Geometry check sheet. Reference: the model listing, model coordinates, mm. A direction names the side the tool comes from. Coordinates: 2 decimals unless noted, no trailing zeros. Order: outer loops, then holes, each group sorted by start corner. A loop starts at its lowest first (then second) coordinate and runs counter-clockwise, first axis right, second up. Notation, with made-up numbers: (5.5, -32) - (21.5, -32) arc R23 ccw to (21.5, -15) - close; hole circle Ø5 at (-37, -9). An arc over 180 degrees is marked (long way). Return JSON: item names as keys, results as strings. Group by question number.
Item 1: Gauge pin test, flat ends, axial feed: pin 1 (4 mm diameter, centred on y = -27, z = 74.5, fed in from +X); pin 2 (0.8 mm diameter, centred on x = -0.5, z = 22.5, fed in from -Y); pin 3 (1 mm diameter, centred on x = -36, z = 43, fed in from -Y). Record the tip position at first contact, or that the pin passes through.
Item 2: Section check B-B on z = 7. Enter the section's corners in (x, y).
Item 3: Scan lines: probe 1 along Z at (x, y) = (-48, -27); probe 2 along X at (y, z) = (-7.5, 62.5); probe 3 along X at (y, z) = (-30, 30.5). Record each from-to range of solid material in increasing order.
Item 4: Tool access check on faces 1 (the cylindrical face through (-2.1, -2.07, 39.44)), 2 (the flat face through (-1, -21.5, 39)), 3 (the flat face through (-28, -1, 0)). Record the directions out of +Z, -Z, +X, -X, +Y, -Y that give a thin tool (end or side, any length) a straight path to the whole face; none if there is none.
Item 5: Section check A-A on y = -16. Enter the section's corners in (x, z).
Item 6: Draft check along Z on faces 4 (the flat face through (-28, -1, 80)), 5 (the cylindrical face through (-48, -25, 7)), 6 (the flat face through (-25, -1.5, 39)). Enter one of: pulls with the +Z half, pulls with the -Z half, needs draft (parallel to the pull), parting line crosses it, or undercut.
Item 7: Section check D-D on z = 25.5. Enter the section's corners in (x, y).
Item 8: Section check C-C on y = -25.5. Enter the section's corners in (x, z).
from build123d import *

# Parameters (mm, degrees)
F1_DEPTH = 80
F2_R     = 2.5
F3_DEPTH = 1.5


with BuildPart() as f1:
    # F0 (on Top) → F1 (new body)
    with BuildSketch(Plane.XY):
        with BuildLine():
            ThreePointArc((0, -2), (-0.585786, -0.585786), (-2, 0))
            Line((-2, 0), (-47, 0))
            ThreePointArc((-47, 0), (-48.414214, -0.585786), (-49, -2))
            Line((-49, -2), (-49, -31.5))
            Line((-49, -31.5), (-47.5, -31.5))
            Line((-47.5, -31.5), (-47.5, -3.5))
            ThreePointArc((-47.5, -3.5), (-46.914214, -2.085786), (-45.5, -1.5))
            Line((-45.5, -1.5), (-3.5, -1.5))
            ThreePointArc((-3.5, -1.5), (-2.085786, -2.085786), (-1.5, -3.5))
            Line((-1.5, -3.5), (-1.5, -21.5))
            Line((-1.5, -21.5), (0, -21.5))
            Line((0, -21.5), (0, -2))
        make_face()
    extrude(amount=F1_DEPTH)

    # F2 (on face) → F3 (cut, through all)
    with BuildSketch(Plane(origin=(-49, 0, 0), x_dir=(0, -1, 0), z_dir=(-1, 0, 0))):
        with Locations((27, 5.5)):
            Circle(F2_R)
        with Locations((27, 74.5)):
            Circle(F2_R)
    extrude(amount=-F3_DEPTH, mode=Mode.SUBTRACT)


solid = f1.part
Computed:
{
 "1": {"pin 1": "passes through", "pin 2": "stops at y = -21.5", "pin 3": "stops at y = -1.5"},
 "2": {"outline": "(-49, -31.5) - (-47.5, -31.5) - (-47.5, -29) - (-49, -29) - close; (-49, -25) - (-47.5, -25) - (-47.5, -3.5) arc R2 cw to (-45.5, -1.5) - (-3.5, -1.5) arc R2 cw to (-1.5, -3.5) - (-1.5, -21.5) - (0, -21.5) - (0, -2) arc R2 ccw to (-2, 0) - (-47, 0) arc R2 ccw to (-49, -2) - close"},
 "3": {"probe 1": "z = 0 to 3, 8 to 72, 77 to 80", "probe 2": "x = -49 to -47.5, -1.5 to 0", "probe 3": "x = -49 to -47.5"},
 "4": {"face 1": "+Z, -Z, -Y", "face 2": "+Z, -Z, +X, -Y", "face 3": "-Z, +X, -X, +Y, -Y"},
 "5": {"outline": "(-49, 0) - (-47.5, 0) - (-47.5, 80) - (-49, 80) - close; (-1.5, 0) - (0, 0) - (0, 80) - (-1.5, 80) - close"},
 "6": {"face 4": "pulls with the +Z half", "face 5": "undercut", "face 6": "needs draft"},
 "7": {"outline": "(-49, -31.5) - (-47.5, -31.5) - (-47.5, -3.5) arc R2 cw to (-45.5, -1.5) - (-3.5, -1.5) arc R2 cw to (-1.5, -3.5) - (-1.5, -21.5) - (0, -21.5) - (0, -2) arc R2 ccw to (-2, 0) - (-47, 0) arc R2 ccw to (-49, -2) - close"},
 "8": {"outline": "(-49, 0) - (-47.5, 0) - (-47.5, 3.5) - (-49, 3.5) - close; (-49, 7.5) - (-47.5, 7.5) - (-47.5, 72.5) - (-49, 72.5) - close; (-49, 76.5) - (-47.5, 76.5) - (-47.5, 80) - (-49, 80) - close"}
}
